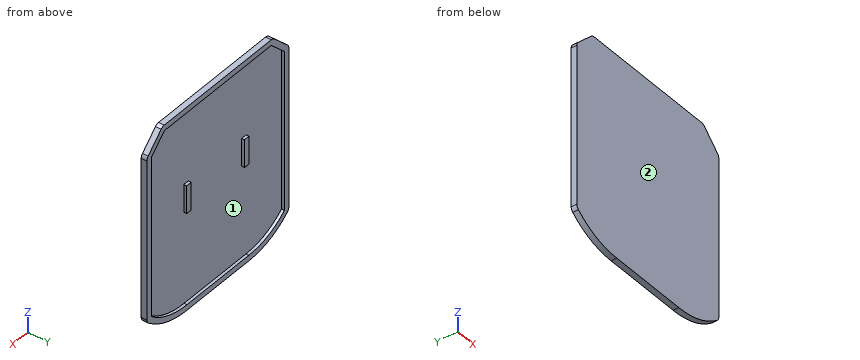
from build123d import *

# Parameters (mm, degrees)
BODY_DEPTH                   = 10
INSIDE_BODY_DEPTH            = 5
SKETCH3_W                    = 10
SKETCH3_H                    = 49.5
HORIZONTAL_CONSTRAINTS_DEPTH = 5
FILLET1_R                    = 10


with BuildPart() as part:
    # Sketch1 → Body (new body)
    with BuildSketch(Plane(origin=(0, 0, 0), x_dir=(1, 0, 0), z_dir=(0, 1, 0))):
        with BuildLine():
            Line((0, 0), (250, 0))
            Line((250, 0), (285.355339059, 35.355339059))
            Line((285.355339059, 35.355339059), (285.355339059, 326.955339059))
            ThreePointArc((285.355339059, 326.955339059), (243.560486982, 353.188356712), (195, 361.955339059))
            Line((195, 361.955339059), (55, 361.955339059))
            ThreePointArc((55, 361.955339059), (6.439513018, 353.188356712), (-35.355339059, 326.955339059))
            Line((-35.355339059, 326.955339059), (-35.355339059, 35.355339059))
            Line((-35.355339059, 35.355339059), (0, 0))
        make_face()
    extrude(amount=BODY_DEPTH)

    # Sketch2 → Inside Body (cut)
    with BuildSketch(Plane(origin=(0, 10, 0), x_dir=(1, 0, 0), z_dir=(0, 1, 0))):
        with BuildLine():
            Line((-25.355339059, 322.508901748), (-25.355339059, 39.497474683))
            Line((-25.355339059, 39.497474683), (4.142135624, 10))
            Line((4.142135624, 10), (245.857864376, 10))
            Line((245.857864376, 10), (275.355339059, 39.497474683))
            Line((275.355339059, 39.497474683), (275.355339059, 322.508901748))
            ThreePointArc((275.355339059, 322.508901748), (237.921386907, 344.627720124), (195.062911656, 351.955339059))
            Line((195.062911656, 351.955339059), (54.937088344, 351.955339059))
            ThreePointArc((54.937088344, 351.955339059), (12.078613093, 344.627720124), (-25.355339059, 322.508901748))
        make_face()
    extrude(amount=-INSIDE_BODY_DEPTH, mode=Mode.SUBTRACT)

    # Sketch3 → Horizontal Constraints (add)
    with BuildSketch(Plane(origin=(0, 5, 0), x_dir=(1, 0, 0), z_dir=(0, 1, 0))):
        with Locations((59.644660941, 164.75)):
            Rectangle(SKETCH3_W, SKETCH3_H)
        with Locations((190.355339059, 164.75)):
            Rectangle(SKETCH3_W, SKETCH3_H)
    extrude(amount=HORIZONTAL_CONSTRAINTS_DEPTH)

    # Fillet1
    fillet1_edges = [part.edges().sort_by_distance(p)[0] for p in [
        (-35.355339059, 5, -326.955339059),
        (285.355339059, 5, -326.955339059),
        (285.355339059, 5, -35.355339059),
        (250, 5, 0),
        (0, 5, 0),
        (-35.355339059, 5, -35.355339059),
    ]]
    fillet(fillet1_edges, radius=FILLET1_R)


solid = part.part
CAD build for the part. Positions are in the model's coordinates, mm. Face numbers are marked on the shaded views. Coordinates: 2 decimals unless noted, no trailing zeros. Write each loop counter-clockwise with the first axis right and the second up, starting at its lowest first coordinate (ties: lowest second). Pieces come first, ordered by that corner, then holes. Notation, with made-up numbers: M 16.5,12.25 L 45.5,12.25 A8 cw 45.5,27.25 Z; hole C 78.5,8 d2. An arc over 180 degrees is marked long. Answer as a JSON object with one key per item and string values. Group by question number.
1) Saw through at C-C (x = 104.5). Write the cut outline in (y, z).
2) Mould opens along X. For the marked faces 1 and 2 say: +X half, -X half, draft (parallel to the pull), parting line (faces both ways), or undercut.
3) Pin check, flat tips, straight feed: pin 1 Ø1.5 at (x, y) = (60, 8) entering from -Z; pin 2 Ø10 at (x, z) = (81.5, -297) entering from +Y. Stop position of each tip, or through.
4) Saw through at B-B (z = -160). Write the cut outline in (x, y).
5) Saw through at D-D (z = -311). Write the cut outline in (x, y).
6) Saw through at A-A (y = 6.75). Give the number of separate pieces and of enclosed holes in the cut face, plus the area to 3 significant figures.
7) Wall check: line 1 (Z direction, x = 59.5, y = 9.5); line 2 (X direction, y = 7, z = -107); line 3 (Y direction, x = 55, z = -105). Give the ranges that are in metal, low to high. Write a range as from..to.
Values follow:
{
 "1": {"outline": "M 0,-361.96 L 10,-361.96 L 10,-351.96 L 5,-351.96 L 5,-10 L 10,-10 L 10,0 L 0,0 Z"},
 "2": {"face 1": "undercut", "face 2": "draft"},
 "3": {"pin 1": "stops at z = -361.96", "pin 2": "stops at y = 5"},
 "4": {"outline": "M -35.36,0 L 285.36,0 L 285.36,10 L 275.36,10 L 275.36,5 L 195.36,5 L 195.36,10 L 185.36,10 L 185.36,5 L 64.64,5 L 64.64,10 L 54.64,10 L 54.64,5 L -25.36,5 L -25.36,10 L -35.36,10 Z"},
 "5": {"outline": "M -35.36,0 L 285.36,0 L 285.36,10 L 275.36,10 L 275.36,5 L -25.36,5 L -25.36,10 L -35.36,10 Z"},
 "6": {"separate pieces": "3", "enclosed holes": "1", "area": "13,400 mm2"},
 "7": {"line 1": "z = -361.96..-351.96, -189.5..-140, -10..0", "line 2": "x = -35.36..-25.36, 275.36..285.36", "line 3": "y = 0..5"}
}
